For this review, take the finished solid that the model builds, in its own axes (mm). A direction names the side the tool comes from. Coordinates: 2 decimals unless noted, no trailing zeros. Write each loop counter-clockwise with the first axis right and the second up, starting at its lowest first coordinate (ties: lowest second). Pieces come first, ordered by that corner, then holes. Notation, with made-up numbers: (34.25, 31) -> (48.25, 31) arc R19 cw to (48.25, 48) -> close; hole circle Ø4 at (32.5, 45.5). An arc over 180 degrees is marked (long way). Put each result on its own line as item: value. Start each with the question number.
Item 1: Consider section D-D on y = -88. Give the boundary of the cut face in (x, z), and give its area (3 significant figures).
Item 2: To check wall thickness, follow L1, parallel to Y at x = 26, z = 83; L2, parallel to X at y = -34.5, z = 28; L3, parallel to Z at x = 56.5, y = -94. State the ranges of each line that lie inside material, in increasing order.
Item 3: Insertion check: P1, Ø15, axis at y = -31, z = 19, coming from the -X side; P2, Ø6, axis at x = 146, y = -63, coming from the +Z side; P3, Ø2, axis at x = 135, z = 11.5, coming from the +Y side; P4, Ø8, axis at x = 29.5, y = -54, coming from the +Z side. Each pin has a flat end and moves straight along its axis. Give the tip position at first contact, or say it passes through.
Item 4: Consider section A-A on y = -35.5. Give the boundary of the cut face in (x, z), and give its area (3 significant figures).
Item 5: Consider section C-C on z = 42. Give the boundary of the cut face in (x, y), and give its area (3 significant figures).
Item 6: Consider section B-B on x = 5.5. Give the boundary of the cut face in (y, z).
Item 7: For faces 1 (the flat face through (51, -25.4, 89)), 2 (the flat face through (90, -76.2, 25)), 3 (the flat face through (0, -38, 25)), 4 (the flat face through (102.38, -40, 70)), 5 (the flat face through (90, -38, 0)), list the 3-axis set-ups (+Z, -Z, +X, -X, +Y, -Y) from which the entire face can be reached by the end or side of a thin tool; tool diameter is ignored.
```python
from build123d import *

# Parameters (mm, degrees)
F0_W     = 203.2
F0_H     = 101.6
F1_DEPTH = 76.2
F2_DEPTH = 50.8
F3_W     = 127
F3_H     = 101.6
F4_DEPTH = 50.8
F5_DEPTH = 25.4
F6_DEPTH = 25.4
F7_W     = 101.6
F7_H     = 76.2
F8_DEPTH = 25.4


with BuildPart() as f1:
    # F0 (on Front) → F1 (new body)
    with BuildSketch(Plane.XZ):
        with Locations((101.6, 50.8)):
            Rectangle(F0_W, F0_H)
    extrude(amount=F1_DEPTH)

    # F2 (cut): a face of the model
    f2_faces = [f1.faces().sort_by_distance(p)[0] for p in [
        (101.6, -38.1, 101.6),
    ]]
    extrude(f2_faces, amount=-F2_DEPTH, mode=Mode.SUBTRACT)

    # F3 (on face) → F4 (join)
    with BuildSketch(Plane.XY.offset(50.8)):
        with Locations((38.8798168193, -50.8)):
            Rectangle(F3_W, F3_H)
    extrude(amount=F4_DEPTH)

    # F5 (add): a face of the model
    f5_faces = [f1.faces().sort_by_distance(p)[0] for p in [
        (203.2, -38.1, 25.4),
    ]]
    extrude(f5_faces, amount=-F5_DEPTH)

    # F6 (cut): a face of the model
    f6_faces = [f1.faces().sort_by_distance(p)[0] for p in [
        (203.2, -38.1, 25.4),
    ]]
    extrude(f6_faces, amount=-F6_DEPTH, mode=Mode.SUBTRACT)

    # F7 (on face) → F8 (cut)
    with BuildSketch(Plane.XY.offset(101.6)):
        with Locations((51.5798168193, -63.5)):
            Rectangle(F7_W, F7_H)
    extrude(amount=-F8_DEPTH, mode=Mode.SUBTRACT)


solid = f1.part
```
Return value:
1. outline: (-24.62, 50.8) -> (102.38, 50.8) -> (102.38, 76.2) -> (0.78, 76.2) -> (0.78, 101.6) -> (-24.62, 101.6) -> close
1. area: 3,870 mm^2
2. L1: -25.4 to 0
2. L2: 0 to 177.8
2. L3: 50.8 to 76.2
3. P1: x = 0
3. P2: z = 50.8
3. P3: y = 0
3. P4: z = 76.2
4. outline: (-24.62, 50.8) -> (0, 50.8) -> (0, 0) -> (177.8, 0) -> (177.8, 50.8) -> (102.38, 50.8) -> (102.38, 76.2) -> (0.78, 76.2) -> (0.78, 101.6) -> (-24.62, 101.6) -> close
4. area: 12,900 mm^2
5. outline: (0, -76.2) -> (177.8, -76.2) -> (177.8, 0) -> (0, 0) -> close
5. area: 13,500 mm^2
6. outline: (-101.6, 50.8) -> (-76.2, 50.8) -> (-76.2, 0) -> (0, 0) -> (0, 101.6) -> (-25.4, 101.6) -> (-25.4, 76.2) -> (-101.6, 76.2) -> close
7. face 1: +Z, +X, -Y
7. face 2: -Z, +X, -X, -Y
7. face 3: -Z, -X, +Y, -Y
7. face 4: +Z, +X, +Y, -Y
7. face 5: -Z, +X, -X, +Y, -Y
